For this review, take the finished solid that the model builds, in its own axes (mm). Face numbers are marked on the shaded views. Coordinates: 2 decimals unless noted, no trailing zeros. Write each loop counter-clockwise with the first axis right and the second up, starting at its lowest first coordinate (ties: lowest second). Pieces come first, ordered by that corner, then holes. Notation, with made-up numbers: (30.5, 29.25) - (54.5, 29.25) arc R27 ccw to (54.5, 52.25) - close; hole circle Ø6 at (32.5, 17). An arc over 180 degrees is marked (long way). Use one line per item in the form item = value. Start each with the question number.
1) We need section A-A (x = -28). Give the boundary of the cut face in (y, z), plus the area to 3 significant figures.
2) Insertion check: P1, Ø2.5, axis at x = 35, z = 7.5, coming from the +Y side. The pin has a flat end and moves straight along its axis. Give the tip position at first contact, or say it passes through.
3) We need section B-B (z = 7.5). Give the boundary of the cut face in (x, y), plus the area to 3 significant figures.
4) Mouldability with a two-part tool opening along X and no side actions: class the marked faces 1, 2, 3 and 4 as pulls with the +X half, pulls with the -X half, needs draft (parallel to the pull), parting line crosses it, or undercut.
5) For L1, parallel to X at y = 2.15, z = 0; L2, parallel to Z at x = -28, y = 3.5; L3, parallel to Z at x = 35, y = 3.25, list the stretches that pass through material, from the lowest coordinate up. Write a range as from..to.
6) We need section D-D (z = 0). Give the boundary of the cut face in (x, y).
7) We need section C-C (y = 3.35). Give the boundary of the cut face in (x, z).
Solid Edge part; units mm, degrees
sketch "Sketch1" plane through (0, 0, 0) normal (0, 1, 0) x (-1, 0, 0)
  line L0 (40, -12.5) -> (-40, -12.5)
  line L1 (-40, -12.5) -> (-40, 12.5)
  line L2 (-40, 12.5) -> (40, 12.5)
  line L3 (40, 12.5) -> (40, -12.5)
  dimension "D1" = 40
  dimension "D2" = 40
extrude "Protrusion1" add sketch "Sketch1" along normal blind 5
hole "Hole_5" at (-28, 5, -0.5) direction (0, -1, 0) diameter 12 end through all
hole "Hole_15" at (35, 0, 7.5) direction (0, 1, 0) diameter 3.2 end through all
hole "Hole1" at (35, 0, -7.5) direction (0, 1, 0) diameter 3.2 end through all
hole "Hole_17" at (-13, 5, 0) direction (0, -1, 0) diameter 3.2 end up to next
hole "Hole2" at (9, 5, 0) direction (0, -1, 0) diameter 3.2 end up to next
properties material "アルミニウム, 5050"
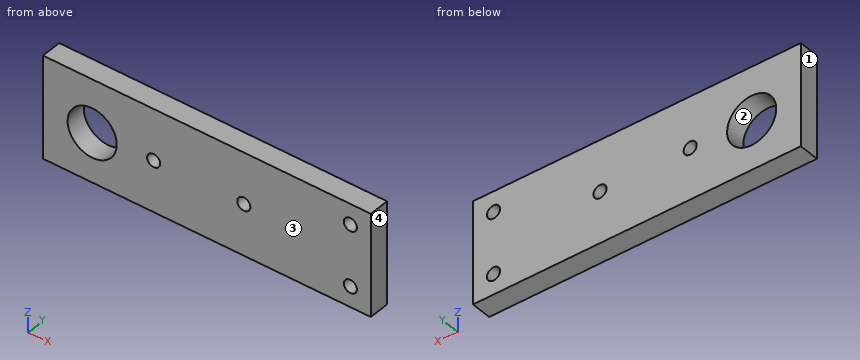
Determined:
q1.outline = (0, -12.5) - (5, -12.5) - (5, -6.5) - (0, -6.5) - close; (0, 5.5) - (5, 5.5) - (5, 12.5) - (0, 12.5) - close
q1.area = 65.0 mm²
q2.P1 = through
q3.outline = (-40, 0) - (33.4, 0) - (33.4, 5) - (-40, 5) - close; (36.6, 0) - (40, 0) - (40, 5) - (36.6, 5) - close
q3.area = 384 mm²
q4.face_1 = pulls with the -X half
q4.face_2 = undercut
q4.face_3 = needs draft
q4.face_4 = pulls with the +X half
q5.L1 = -40..-33.98, -22.02..-14.6, -11.4..7.4, 10.6..40
q5.L2 = -12.5..-6.5, 5.5..12.5
q5.L3 = -12.5..-9.1, -5.9..5.9, 9.1..12.5
q6.outline = (-40, 0) - (-33.98, 0) - (-33.98, 5) - (-40, 5) - close; (-22.02, 0) - (-14.6, 0) - (-14.6, 5) - (-22.02, 5) - close; (-11.4, 0) - (7.4, 0) - (7.4, 5) - (-11.4, 5) - close; (10.6, 0) - (40, 0) - (40, 5) - (10.6, 5) - close
q7.outline = (-40, -12.5) - (40, -12.5) - (40, 12.5) - (-40, 12.5) - close; hole circle Ø12 at (-28, -0.5); hole circle Ø3.2 at (-13, 0); hole circle Ø3.2 at (9, 0); hole circle Ø3.2 at (35, -7.5); hole circle Ø3.2 at (35, 7.5)
